For this review, use the dimensioned drawing (mm, ordinates from the lowest corner) and the shaded views. A direction names the side the tool comes from. Coordinates: 2 decimals unless noted, no trailing zeros. Loops run counter-clockwise (first coordinate to the right, second up) from the corner with the lowest first, then second, coordinate; pieces in that order, holes last. Notation, with made-up numbers: M 33.5,2.5 L 90.5,2.5 A14 cw 90.5,24.5 Z; hole C -3.75,85 d5. An arc over 180 degrees is marked long. Write item = value, one per line.
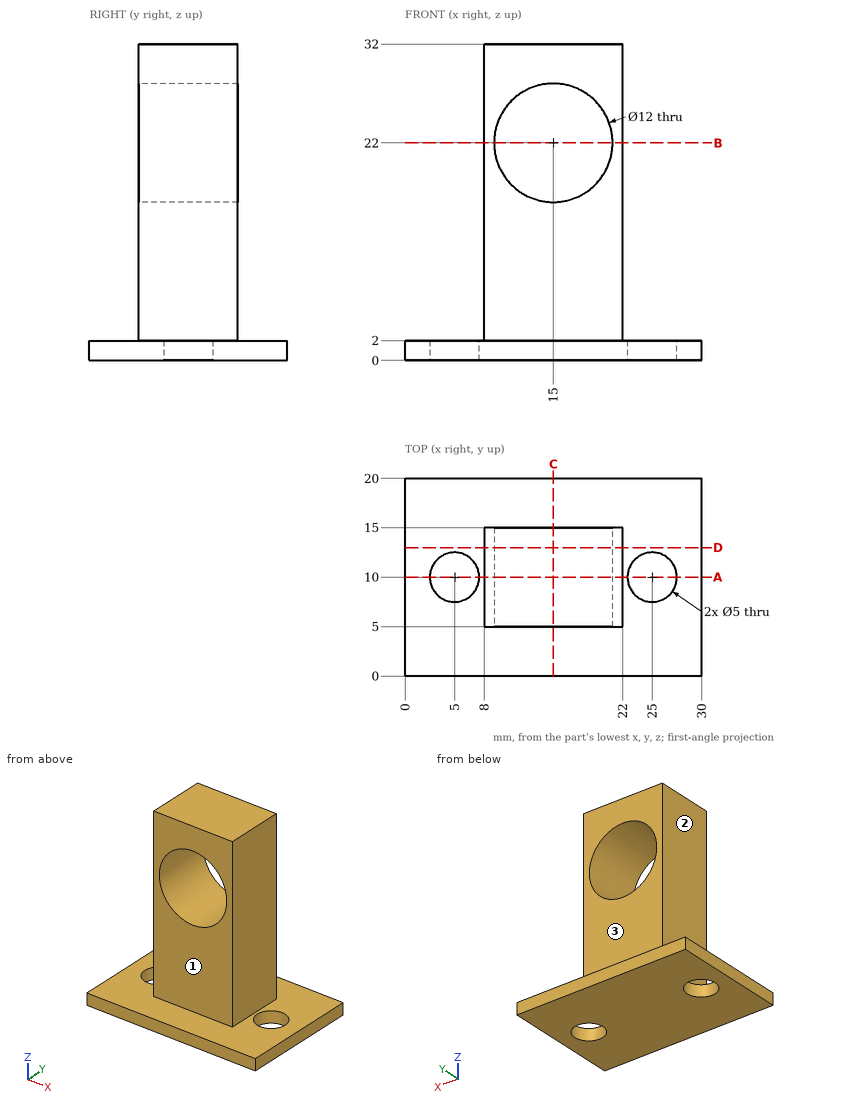
Q1. For line 1 along Z through (x, y) = (15, 13); line 2 along Y through (x, z) = (25, 0.7); line 3 along Z through (x, y) = (10.75, 15.25), list the stretches that pass through material, from the lowest coordinate up.
Solved:
line_1 = 0 to 16, 28 to 32
line_2 = 0 to 7.5, 12.5 to 20
line_3 = 0 to 2
Q2. Add section D-D (y = 13). Write out the cut boundary in (x, z), and give its area (3 significant figures).
Solved:
outline = M 0,0 L 30,0 L 30,2 L 22,2 L 22,32 L 8,32 L 8,2 L 0,2 Z; hole C 15,22 d12
area = 367 mm²
Q3. For pin 1 Ø11 at (x, z) = (16, 12) entering from -Y; pin 2 Ø3 at (y, z) = (16, 13.5) entering from +X; pin 3 Ø2 at (y, z) = (17.5, 13) entering from +X; pin 4 Ø1.5 at (y, z) = (15.5, 27) entering from -X, all flat-tipped, find the tip position at first contact; note any pin that passes through.
Solved:
pin_1 = 5
pin_2 = 22
pin_3 = through
pin_4 = 8
Q4. Add section A-A (y = 10). Write out the cut boundary in (x, z).
Solved:
outline = M 0,0 L 2.5,0 L 2.5,2 L 0,2 Z; M 7.5,0 L 22.5,0 L 22.5,2 L 22,2 L 22,32 L 8,32 L 8,2 L 7.5,2 Z; M 27.5,0 L 30,0 L 30,2 L 27.5,2 Z; hole C 15,22 d12
Q5. Add section C-C (x = 15). Write out the cut boundary in (y, z), and give its area (3 significant figures).
Solved:
outline = M 0,0 L 20,0 L 20,2 L 15,2 L 15,16 L 5,16 L 5,2 L 0,2 Z; M 5,28 L 15,28 L 15,32 L 5,32 Z
area = 220 mm²
Q6. Add section B-B (z = 22). Write out the cut boundary in (x, y), and give its area (3 significant figures).
Solved:
outline = M 8,5 L 9,5 L 9,15 L 8,15 Z; M 21,5 L 22,5 L 22,15 L 21,15 Z
area = 20.0 mm²
Q7. Machinability: for the marked faces 1, 2 and 3, which of the approach directions +Z, -Z, +X, -X, +Y, -Y give a long, thin tool a straight path to every point of the face, cutting with its end or side? Answer none if there is none.
Solved:
face_1 = +Z, +X, -X, -Y
face_2 = +Z, -X, +Y, -Y
face_3 = +Z, +X, -X, +Y
